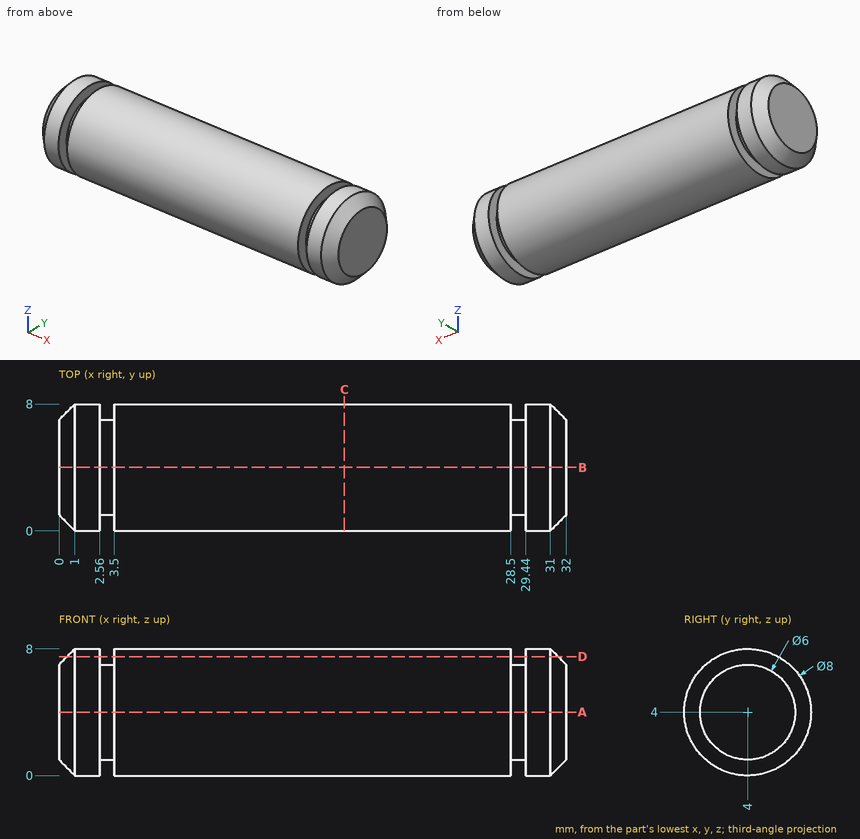
Could you check a few things on this drawing? It's one solid part, dimensions in mm from its lowest x, y, z. Round coordinates to 2 decimals unless told otherwise and drop trailing zeros. Write each loop counter-clockwise with the first axis right and the second up, starting at its lowest first coordinate (ties: lowest second). Pieces come first, ordered by that corner, then holes. Notation, with made-up numbers: (24.5, 88.5) -> (47.5, 88.5) arc R20 cw to (47.5, 110.5) -> close; hole circle Ø3 at (56, -19.75). An arc over 180 degrees is marked (long way). One line per question, with ' | ' between items. Start each with the question number.
1) Suppose I cut it at D-D on z = 7.5. Count the separate pieces of the cut face and the enclosed holes in it, then the cut area to 3 significant figures.
2) Suppose I cut it at A-A on z = 4. Write out the boundary of the cut face in (x, y), then the cut area to 3 significant figures.
3) I need wall thicknesses on line 1 (X direction, y = 7.25, z = 4.5); line 2 (X direction, y = 3.25, z = 7); line 3 (Z direction, x = 24, y = 3.5). Which ranges of each line are inside material? Lowest first, please. Write a range as [from, to].
4) Suppose I cut it at C-C on x = 18. Write out the boundary of the cut face in (y, z).
5) I'm going to push a flat-ended pin straight in: P1, Ø1, axis at x = 17.5, z = 1.5, coming from the +Y side. Where does the tip first touch, or does it pass through?
Return value:
1) separate pieces: 3 | enclosed holes: 0 | area: 111 mm2
2) outline: (0, 1) -> (1, 0) -> (2.56, 0) -> (2.56, 1) -> (3.5, 1) -> (3.5, 0) -> (28.5, 0) -> (28.5, 1) -> (29.44, 1) -> (29.44, 0) -> (31, 0) -> (32, 1) -> (32, 7) -> (31, 8) -> (29.44, 8) -> (29.44, 7) -> (28.5, 7) -> (28.5, 8) -> (3.5, 8) -> (3.5, 7) -> (2.56, 7) -> (2.56, 8) -> (1, 8) -> (0, 7) -> close | area: 250 mm2
3) line 1: x = [0.29, 2.56], [3.5, 28.5], [29.44, 31.71] | line 2: x = [0.09, 2.56], [3.5, 28.5], [29.44, 31.91] | line 3: z = [0.03, 7.97]
4) outline: circle Ø8 at (4, 4)
5) P1: stops at y = 7.46
